The listing builds one solid part. Answer for the finished solid, in the listing's coordinates (mm). A direction names the side the tool comes from. Coordinates: 2 decimals unless noted, no trailing zeros. Order: outer loops, then holes, each group sorted by start corner. A loop starts at its lowest first (then second) coordinate and runs counter-clockwise, first axis right, second up. Notation, with made-up numbers: (59, 30.25) -> (71, 30.25) arc R30 ccw to (71, 68.25) -> close; hole circle Ø10 at (29, 72). An arc over 180 degrees is marked (long way). Answer in a Markdown table with one row per item.
```python
from build123d import *

# Parameters (mm, degrees)
ESQUISSE1_W        = 20
ESQUISSE1_H        = 10
BOSS_EXTRU_1_DEPTH = 500
ESQUISSE2_W        = 30
ESQUISSE2_H        = 15
BOSS_EXTRU_2_DEPTH = 10


with BuildPart() as part:
    # Esquisse1 → Boss.-Extru.1 (new body)
    with BuildSketch(Plane.XY):
        Rectangle(ESQUISSE1_W, ESQUISSE1_H)
    boss_extru_1 = extrude(amount=BOSS_EXTRU_1_DEPTH)

    # Esquisse2 → Boss.-Extru.2 (add)
    with BuildSketch(Plane.XY.offset(500)):
        Rectangle(ESQUISSE2_W, ESQUISSE2_H)
    boss_extru_2 = extrude(amount=BOSS_EXTRU_2_DEPTH)

    # Symétrie1: Boss.-Extru.1, Boss.-Extru.2 across plane
    add(boss_extru_1.mirror(Plane.XY))
    add(boss_extru_2.mirror(Plane.XY))


solid = part.part
```
(1) A cutting plane is placed at C-C, the plane z = 232.5. Determine the outline of the cut face in (x, y), then the cut area to 3 significant figures.
Check values:
| item | result |
|---|---|
| outline | (-10, -5) -> (10, -5) -> (10, 5) -> (-10, 5) -> close |
| area | 200 mm² |
(2) A cutting plane is placed at A-A, the plane y = 2.5. Determine the outline of the cut face in (x, z), then the cut area to 3 significant figures.
Check values:
| item | result |
|---|---|
| outline | (-15, -510) -> (15, -510) -> (15, -500) -> (10, -500) -> (10, 500) -> (15, 500) -> (15, 510) -> (-15, 510) -> (-15, 500) -> (-10, 500) -> (-10, -500) -> (-15, -500) -> close |
| area | 20,600 mm² |
(3) Which of the six approach directions +Z, -Z, +X, -X, +Y, -Y give full straight-line access (tool end or side, diameter ignored) to faces 1 (the flat face through (0, -5, 7)), 2 (the flat face through (0, 5, 7))?
Check values:
| item | result |
|---|---|
| face 1 | +X, -X, -Y |
| face 2 | +X, -X, +Y |
(4) Flat-ended cylindrical pins translate along their axes: pin 1 (5 mm diameter, centred on x = 3.5, z = -32.5, fed in from -Y); pin 2 (3 mm diameter, centred on y = 2, z = 72.5, fed in from +X); pin 3 (1 mm diameter, centred on y = 0, z = 373.5, fed in from -X). Find the tip coordinate at first contact, or state that the pin passes through.
Check values:
| item | result |
|---|---|
| pin 1 | y = -5 |
| pin 2 | x = 10 |
| pin 3 | x = -10 |
(5) A cutting plane is placed at B-B, the plane x = 4.25. Determine the outline of the cut face in (y, z).
Check values:
| item | result |
|---|---|
| outline | (-7.5, -510) -> (7.5, -510) -> (7.5, -500) -> (5, -500) -> (5, 500) -> (7.5, 500) -> (7.5, 510) -> (-7.5, 510) -> (-7.5, 500) -> (-5, 500) -> (-5, -500) -> (-7.5, -500) -> close |
(6) Find the intervals of material crossed by line 1 along Z through (x, y) = (1.25, -6.5); line 2 along Y through (x, z) = (-3.25, -377); line 3 along X through (y, z) = (-1, -356), in increasing order. Write a range as from..to.
Check values:
| item | result |
|---|---|
| line 1 | -510..-500, 500..510 |
| line 2 | -5..5 |
| line 3 | -10..10 |
